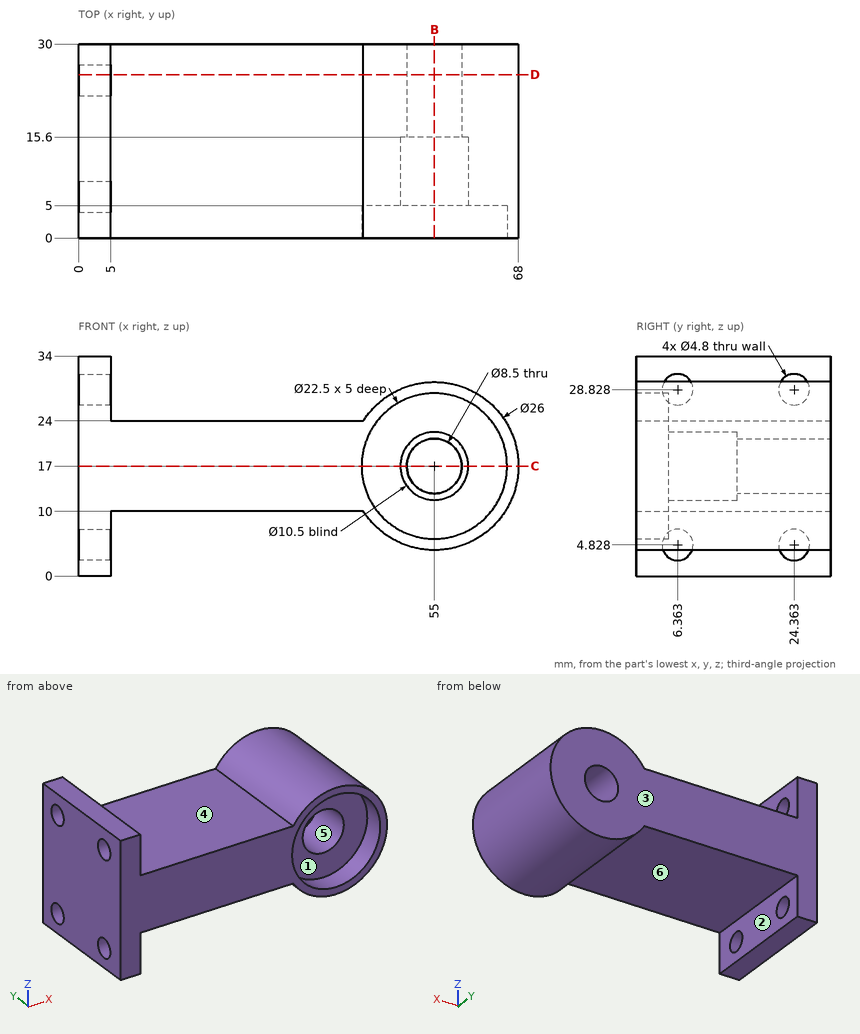
Drawing for the job (mm, zero at the part's lowest x, y, z). A direction names the side the tool comes from. Give positions to 0.01 mm unless a question says otherwise; leave off trailing zeros. Loops run counter-clockwise (first coordinate to the right, second up) from the corner with the lowest first, then second, coordinate; pieces in that order, holes last.
Item 1: Drill centre lines: line 1 along X through (y, z) = (1.75, 8); line 2 along Z through (x, y) = (39.5, 16); line 3 along X through (y, z) = (15.5, 6) (1 decimal). Where is each one in solid material? Low to high.
Check values:
line 1: x = 0 to 5, 45.62 to 48.25, 61.75 to 64.38
line 2: z = 10 to 24
line 3: x = 0 to 5, 48.1 to 61.9
Item 2: Drop flat-ended pins along their axis: P1, Ø4.5, axis at y = 24.36, z = 28.83, coming from the -X side; P2, Ø7.5, axis at y = 6.36, z = 4.83, coming from the +X side (1 decimal); P3, Ø9, axis at x = 21, y = 13, coming from the -Z side; P4, Ø6, axis at y = 6.5, z = 23.5, coming from the -X side. Give the stop position or say it passes through.
Check values:
P1: stops at x = 46.21
P2: stops at x = 64.9
P3: stops at z = 10
P4: stops at x = 0
Item 3: Slice it at D-D (y = 25.25). Give the number of separate pieces and of enclosed holes in the cut face, plus the area to 3 significant figures.
Check values:
separate pieces: 3
enclosed holes: 1
area: 1,130 mm2
Item 4: Mould opens along Z. For the marked faces 4, 5 and 6 say: +Z half, -Z half, draft (parallel to the pull), parting line (faces both ways), or undercut.
Check values:
face 4: +Z half
face 5: undercut
face 6: -Z half
Item 5: Slice it at B-B (x = 55). Write the cut outline in (y, z).
Check values:
outline: (0, 4) - (30, 4) - (30, 12.75) - (15.6, 12.75) - (15.6, 11.75) - (5, 11.75) - (5, 5.75) - (0, 5.75) - close; (0, 28.25) - (5, 28.25) - (5, 22.25) - (15.6, 22.25) - (15.6, 21.25) - (30, 21.25) - (30, 30) - (0, 30) - close
Item 6: Slice it at C-C (z = 17). Write the cut outline in (x, y).
Check values:
outline: (0, 0) - (43.75, 0) - (43.75, 5) - (49.75, 5) - (49.75, 15.6) - (50.75, 15.6) - (50.75, 30) - (0, 30) - close; (59.25, 15.6) - (60.25, 15.6) - (60.25, 5) - (66.25, 5) - (66.25, 0) - (68, 0) - (68, 30) - (59.25, 30) - close
Item 7: Which spindle directions (+Z, -Z, +X, -X, +Y, -Y) get a long thin tool onto all of the face, cutting with end or side? Do the marked faces 1, 2 and 3. Say none if no direction does.
Check values:
face 1: -Y
face 2: -Z, +Y, -Y
face 3: +Z, -Z, +X, -X, +Y
